Autodesk Inventor part; units mm, degrees
ref_plane "YZ Plane" through (0, 0, 0) normal (1, 0, 0) x (0, 1, 0)
ref_plane "XZ Plane" through (0, 0, 0) normal (0, 1, 0) x (-1, 0, 0)
ref_plane "XY Plane" through (0, 0, 0) normal (0, 0, 1) x (1, 0, 0)
sketch "Sketch1" plane through (0, 0, 0) normal (0, 0, 1) x (1, 0, 0)
  arc A0 (0, 0) -> (22, 22) centre (0, 22) ccw
  line L0 (22, 22) -> (22, 37)
  arc A1 (22, 37) -> (13, 54.7482) centre (0, 37) ccw
  line L1 (13, 54.7482) -> (13, 54.7482)
  line L2 (8, 70) -> (23, 70)
  line L3 (40, 62) -> (31.8, 62)
  line L4 (31.8, 62) -> (31.8, 53.8)
  line L5 (31.8, 53.8) -> (40, 53.8)
  line L6 (40, 45.8) -> (31.8, 45.8)
  line L7 (31.8, 45.8) -> (31.8, 37.6)
  line L8 (31.8, 37.6) -> (40, 37.6)
  line L9 (40, 53.8) -> (40, 45.8)
  line L10 (40, 37.6) -> (40, 0)
  line L11 (40, 62) -> (40, 70)
  line L12 (40, 70) -> (23, 70)
  line L13 (23, 70) -> (23, 70)
  line L14 (8, 70) -> (8, 54.7482)
  line L15 (8, 54.7482) -> (13, 54.7482)
  line L16 (0, 0) -> (40, 0)
  point P0 (40, 66)
  dimension "d0" = 22
  dimension "d1" = 90
  dimension "d2" = 0
  dimension "d3" = 15
  dimension "d4" = 0
  dimension "d5" = 13
  dimension "d6" = 22
  dimension "d7" = 0
  dimension "d14" = 8.2
  dimension "d15" = 8.2
  dimension "d32" = 8
  dimension "d34" = 8
  dimension "d35" = 8
  dimension "d37" = 15
  dimension "d39" = 40
  dimension "d40" = 0
  dimension "d41" = 0
  dimension "d42" = 0
  dimension "d43" = 8.2
  dimension "d44" = 70
extrude "Extrusion2" add sketch "Sketch1" along normal blind 8
properties part number "CenterFinger"
Design review of the part built by this model. Coordinates are the model's own, in mm. A direction names the side the tool comes from. Give positions to 0.01 mm unless a question says otherwise; leave off trailing zeros. Order: outer loops, then holes, each group sorted by start corner. A loop starts at its lowest first (then second) coordinate and runs counter-clockwise, first axis right, second up.
1. Add section B-B, the plane z = 7. State the section outline as (x, y) points.
Solution:
outline: (0, 0) - (40, 0) - (40, 37.6) - (31.8, 37.6) - (31.8, 45.8) - (40, 45.8) - (40, 53.8) - (31.8, 53.8) - (31.8, 62) - (40, 62) - (40, 70) - (8, 70) - (8, 54.75) - (13, 54.75) arc R22 cw to (22, 37) - (22, 22) arc R22 cw to start
2. Mouldability with a two-part tool opening along Y and no side actions: class faces 4 (the cylindrical face through (19.556, 47.079, 3.944)), 5 (the flat face through (40, 50, 4)), 6 (the flat face through (36, 45.8, 4)), 7 (the flat face through (20, 0, 4)) as +Y half, -Y half, draft (parallel to the pull), parting line (faces both ways), or undercut.
Solution:
face 4: undercut
face 5: draft
face 6: undercut
face 7: -Y half
3. Tool access review of faces 1 (the flat face through (8, 62, 4)), 2 (the cylindrical face through (15.73, 6.62, 3.94)), 3 (the flat face through (36, 62, 4)): name each direction out of +Z, -Z, +X, -X, +Y, -Y from which nothing blocks a thin tool from reaching the whole face with its end or side.
Solution:
face 1: +Z, -Z, -X, +Y
face 2: +Z, -Z, -X
face 3: +Z, -Z, +X
4. For pin 1 Ø2.5 at (y, z) = (30, 4) entering from -X; pin 2 Ø2.5 at (y, z) = (42, 4.5) entering from +X; pin 3 Ø4 at (y, z) = (44, 1.5) entering from -X, all flat-tipped, find the tip position at first contact; note any pin that passes through.
Solution:
pin 1: stops at x = 22
pin 2: stops at x = 31.8
pin 3: stops at x = 20.07
5. Add section D-D, the plane y = 26.5. State the section outline as (x, z) points, then the cut area to 3 significant figures.
Solution:
outline: (22, 0) - (40, 0) - (40, 8) - (22, 8) - close
area: 144 mm2
6. Add section A-A, the plane x = 37.5. State the section outline as (y, z) points, then the cut area to 3 significant figures.
Solution:
outline: (0, 0) - (37.6, 0) - (37.6, 8) - (0, 8) - close; (45.8, 0) - (53.8, 0) - (53.8, 8) - (45.8, 8) - close; (62, 0) - (70, 0) - (70, 8) - (62, 8) - close
area: 429 mm2
7. To check wall thickness, follow L1, parallel to Y at x = 36.5, z = 3.75; L2, parallel to X at y = 59, z = 3.5; L3, parallel to X at y = 35.5, z = 6. State the ranges of each line that lie inside material, in increasing order.
Solution:
L1: y = 0 to 37.6, 45.8 to 53.8, 62 to 70
L2: x = 8 to 31.8
L3: x = 22 to 40
8. Add section C-C, the plane x = 17. State the section outline as (y, z) points, then the cut area to 3 significant figures.
Solution:
outline: (0, 0) - (8.04, 0) - (8.04, 8) - (0, 8) - close; (50.96, 0) - (70, 0) - (70, 8) - (50.96, 8) - close
area: 217 mm2
